Here's how the part is built. I have some questions about the finished solid (model axes, mm). Give positions to 0.01 mm unless a question says otherwise; leave off trailing zeros. Write each loop counter-clockwise with the first axis right and the second up, starting at its lowest first coordinate (ties: lowest second). Pieces come first, ordered by that corner, then holes. Notation, with made-up numbers: (86.5, 36.5) -> (106.5, 36.5) arc R21 cw to (106.5, 57.5) -> close; hole circle Ø8 at (-37.5, 6.5). An arc over 180 degrees is marked (long way). Use one line per item in the form item = value.
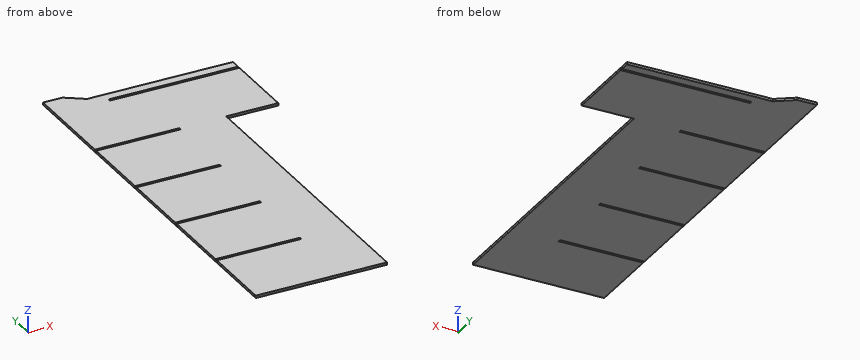
```python
from build123d import *

# Parameters (mm, degrees)
BOSS_EXTRUDE2_DEPTH = 3.175
SKETCH2_W           = 24.39416
SKETCH2_H           = 495.5921
BOSS_EXTRUDE3_DEPTH = 3.175
BOSS_EXTRUDE4_DEPTH = 3.175
SKETCH4_W           = 68.31584
SKETCH4_H           = 12.7
SKETCH4_H_2         = 96.57842
BOSS_EXTRUDE5_DEPTH = 3.175


with BuildPart() as part:
    # Sketch1 → Boss-Extrude2 (new body)
    with BuildSketch(Plane.XY):
        Polygon((129.013076168, 254.245404572), (-18.685383832, 254.245404572), (-18.685383832, 157.666984572), (92.088461168, 157.666984572), (92.088461168, 154.491984572), (-18.685383832, 154.491984572), (-18.685383832, 57.913564572), (92.088461168, 57.913564572), (92.088461168, 54.738564572), (-18.685383832, 54.738564572), (-18.685383832, -41.839855428), (92.088461168, -41.839855428), (92.088461168, -45.014855428), (-18.685383832, -45.014855428), (-18.685383832, -141.593275428), (92.088461168, -141.593275428), (92.088461168, -144.768275428), (-18.685383832, -144.768275428), (-18.685383832, -241.346695428), (129.013076168, -241.346695428), align=None)
    extrude(amount=BOSS_EXTRUDE2_DEPTH)

    # Sketch2 → Boss-Extrude3 (add, through all)
    with BuildSketch(Plane.XY.offset(3.175)):
        with Locations((141.210156168, 6.449354572)):
            Rectangle(SKETCH2_W, SKETCH2_H)
    extrude(amount=-BOSS_EXTRUDE3_DEPTH)

    # Sketch3 → Boss-Extrude4 (add, through all)
    with BuildSketch(Plane.XY.offset(3.175)):
        Polygon((51.807236168, 257.420404572), (51.807236168, 254.245404572), (-18.685383832, 254.245404572), (-18.685383832, 286.376404572), (6.714616168, 286.376404572), (30.496305109, 270.120404572), (153.407236168, 270.120404572), (153.407236168, 257.420404572), align=None)
    extrude(amount=-BOSS_EXTRUDE4_DEPTH)

    # Sketch4 → Boss-Extrude5 (add, through all)
    with BuildSketch(Plane.XY.offset(3.175)):
        with Locations((187.565156168, 263.770404572)):
            Rectangle(SKETCH4_W, SKETCH4_H)
        with Locations((187.565156168, 205.956194572)):
            Rectangle(SKETCH4_W, SKETCH4_H_2)
    extrude(amount=-BOSS_EXTRUDE5_DEPTH)


solid = part.part
```
Q1. I want a section at B-B, the plane x = 46.5. Write out the boundary of the cut face in (y, z) (3 decimals), and give its area (3 significant figures).
Result set:
outline = (-241.347, 0) -> (-144.768, 0) -> (-144.768, 3.175) -> (-241.347, 3.175) -> close; (-141.593, 0) -> (-45.015, 0) -> (-45.015, 3.175) -> (-141.593, 3.175) -> close; (-41.84, 0) -> (54.739, 0) -> (54.739, 3.175) -> (-41.84, 3.175) -> close; (57.914, 0) -> (154.492, 0) -> (154.492, 3.175) -> (57.914, 3.175) -> close; (157.667, 0) -> (270.12, 0) -> (270.12, 3.175) -> (157.667, 3.175) -> close
area = 1,580 mm2
Q2. I want a section at A-A, the plane x = 207.5. Write out the boundary of the cut face in (y, z) (3 decimals), and give its area (3 significant figures).
Result set:
outline = (157.667, 0) -> (254.245, 0) -> (254.245, 3.175) -> (157.667, 3.175) -> close; (257.42, 0) -> (270.12, 0) -> (270.12, 3.175) -> (257.42, 3.175) -> close
area = 347 mm2
Q3. I want a section at D-D, the plane x = 118.5. Write out the boundary of the cut face in (y, z) (3 decimals), and give its area (3 significant figures).
Result set:
outline = (-241.347, 0) -> (254.245, 0) -> (254.245, 3.175) -> (-241.347, 3.175) -> close; (257.42, 0) -> (270.12, 0) -> (270.12, 3.175) -> (257.42, 3.175) -> close
area = 1,610 mm2
Q4. I want a section at C-C, the plane z = 2.3. Write out the boundary of the cut face in (x, y).
Result set:
outline = (-18.69, -241.35) -> (153.41, -241.35) -> (153.41, 157.67) -> (221.72, 157.67) -> (221.72, 254.25) -> (51.81, 254.25) -> (51.81, 257.42) -> (221.72, 257.42) -> (221.72, 270.12) -> (30.5, 270.12) -> (6.71, 286.38) -> (-18.69, 286.38) -> (-18.69, 157.67) -> (92.09, 157.67) -> (92.09, 154.49) -> (-18.69, 154.49) -> (-18.69, 57.91) -> (92.09, 57.91) -> (92.09, 54.74) -> (-18.69, 54.74) -> (-18.69, -41.84) -> (92.09, -41.84) -> (92.09, -45.01) -> (-18.69, -45.01) -> (-18.69, -141.59) -> (92.09, -141.59) -> (92.09, -144.77) -> (-18.69, -144.77) -> close
Q5. If I drill on line 1 along Y through (x, z) = (-0.5, 2.95); line 2 along Y through (x, z) = (68, 1.8); line 3 along Y through (x, z) = (198, 0.25), over which ranges is the centre line in solid material (lowest first)? Write a range as from..to.
Result set:
line_1 = -241.35..-144.77, -141.59..-45.01, -41.84..54.74, 57.91..154.49, 157.67..286.38
line_2 = -241.35..-144.77, -141.59..-45.01, -41.84..54.74, 57.91..154.49, 157.67..254.25, 257.42..270.12
line_3 = 157.67..254.25, 257.42..270.12
Q6. Will these pins go through, and if not, where does the flat tip stop? pin 1 Ø1.6 at (x, z) = (26.5, 1) entering from +Y; pin 2 Ø1.6 at (y, z) = (255.5, 1) entering from +X; pin 3 Ø1 at (x, z) = (46, 2) entering from +Y.
Result set:
pin_1 = 273.4
pin_2 = 51.81
pin_3 = 270.12
